Verification items for the finished model (mm, model axes). A direction names the side the tool comes from. Round coordinates to 2 decimals unless told otherwise and drop trailing zeros. Loops run counter-clockwise (first coordinate to the right, second up) from the corner with the lowest first, then second, coordinate; pieces in that order, holes last. Notation, with made-up numbers: (69, -27.5) - (83, -27.5) arc R13 cw to (83, -13.5) - close; hole circle Ø10 at (40.5, 65). An arc over 180 degrees is marked (long way). Use a Markdown table: item, result. Add a question column.
Autodesk Inventor part; units mm, degrees
ref_plane "YZ Plane" through (0, 0, 0) normal (1, 0, 0) x (0, 1, 0)
ref_plane "XZ Plane" through (0, 0, 0) normal (0, 1, 0) x (-1, 0, 0)
ref_plane "XY Plane" through (0, 0, 0) normal (0, 0, 1) x (1, 0, 0)
sketch "Sketch1" plane through (0, 0, 0) normal (0, 0, 1) x (1, 0, 0)
  line L0 (0, 0) -> (44.45, 0)
  line L1 (44.45, 0) -> (44.45, 44.45)
  line L2 (44.45, 44.45) -> (19.05, 44.45)
  line L3 (19.05, 44.45) -> (19.05, 25.4)
  line L4 (19.05, 25.4) -> (0, 25.4)
  line L5 (0, 25.4) -> (0, 0)
  circle A0 centre (6.35, 12.7) radius 2.0701
  circle A1 centre (31.75, 12.7) radius 2.0701
  circle A2 centre (31.75, 38.1) radius 2.0701
  dimension "d0" = 44.45
  dimension "d1" = 25.4
  dimension "d2" = 4.1402
  dimension "d3" = 12.7
  dimension "d4" = 6.35
  dimension "d7" = 25.4
  dimension "d14" = 25.4
extrude "Extrusion1" add sketch "Sketch1" along normal blind 6.35
fillet "Fillet1" radius 3.175 6 edges at (19.05, 25.4, 3.175) (0, 25.4, 3.175) (0, 0, 3.175) (44.45, 0, 3.175) (44.45, 44.45, 3.175) (19.05, 44.45, 3.175)
properties part number "Spacer 2" material "ABS Plastic"
Q1. Section check D-D on y = 12.7. Record the cut outline in (x, z).
Q2. Section check A-A on y = 38.1. Record the cut outline in (x, z), plus the area to 3 significant figures.
Q3. Section check C-C on z = 5.75. Record the cut outline in (x, y) (3 decimals).
Q4. Go/stop test with flat-tipped pins: pin 1 Ø8 at (x, y) = (13, 34.5) entering from +Z; pin 2 Ø6.5 at (x, y) = (6.35, 12.7) entering from -Z; pin 3 Ø3 at (x, z) = (8, 4) entering from +Y; pin 4 Ø1.5 at (y, z) = (26.5, 2) entering from -X. Record where each tip stops, or that it passes through.
Q5. Section check B-B on x = 31.75. Record the cut outline in (y, z), plus the area to 3 significant figures.
Q6. Release check for a two-part mould opening along Y. For faces 3 (the face through (44.45, 22, 3)), 4 (the face through (0.91, 0.95, 3.22)), 5 (the face through (29.68, 12.61, 3.13)), 6 (the face through (6.081, 10.648, 3.131)) record: +Y half, -Y half, draft (parallel to the pull), parting line (faces both ways), or undercut.
Q7. Thickness scan on line 1 along X through (y, z) = (12.5, 1); line 2 along Y through (x, z) = (31.75, 2.5); line 3 along Y through (x, z) = (6.35, 4.5). Record the ranges inside material, lowest first.
Q8. Set-up check for faces 1 (the face through (0, 13, 3)), 2 (the face through (19.05, 35, 3)): record each of +Z, -Z, +X, -X, +Y, -Y from which the full face is reachable in a straight line by a thin tool's end or side.
Determined:
| question | item | result |
|---|---|---|
| 1 | outline | (0, 0) - (4.28, 0) - (4.28, 6.35) - (0, 6.35) - close; (8.42, 0) - (29.68, 0) - (29.68, 6.35) - (8.42, 6.35) - close; (33.82, 0) - (44.45, 0) - (44.45, 6.35) - (33.82, 6.35) - close |
| 2 | outline | (19.05, 0) - (29.68, 0) - (29.68, 6.35) - (19.05, 6.35) - close; (33.82, 0) - (44.45, 0) - (44.45, 6.35) - (33.82, 6.35) - close |
| 2 | area | 135 mm² |
| 3 | outline | (0, 3.175) arc R3.175 ccw to (3.175, 0) - (41.275, 0) arc R3.175 ccw to (44.45, 3.175) - (44.45, 41.275) arc R3.175 ccw to (41.275, 44.45) - (22.225, 44.45) arc R3.175 ccw to (19.05, 41.275) - (19.05, 28.575) arc R3.175 cw to (15.875, 25.4) - (3.175, 25.4) arc R3.175 ccw to (0, 22.225) - close; hole circle Ø4.14 at (6.35, 12.7); hole circle Ø4.14 at (31.75, 12.7); hole circle Ø4.14 at (31.75, 38.1) |
| 4 | pin 1 | passes through |
| 4 | pin 2 | stops at z = 0 |
| 4 | pin 3 | stops at y = 25.4 |
| 4 | pin 4 | stops at x = 17.32 |
| 5 | outline | (0, 0) - (10.63, 0) - (10.63, 6.35) - (0, 6.35) - close; (14.77, 0) - (36.03, 0) - (36.03, 6.35) - (14.77, 6.35) - close; (40.17, 0) - (44.45, 0) - (44.45, 6.35) - (40.17, 6.35) - close |
| 5 | area | 230 mm² |
| 6 | face 3 | draft |
| 6 | face 4 | -Y half |
| 6 | face 5 | undercut |
| 6 | face 6 | undercut |
| 7 | line 1 | x = 0 to 4.29, 8.41 to 29.69, 33.81 to 44.45 |
| 7 | line 2 | y = 0 to 10.63, 14.77 to 36.03, 40.17 to 44.45 |
| 7 | line 3 | y = 0 to 10.63, 14.77 to 25.4 |
| 8 | face 1 | +Z, -Z, -X, +Y, -Y |
| 8 | face 2 | +Z, -Z, -X, +Y |
